Read the model definition and answer for the solid it produces. Units are mm, in the model's axes. A direction names the side the tool comes from. Round coordinates to 2 decimals unless told otherwise and drop trailing zeros. Write each loop counter-clockwise with the first axis right and the second up, starting at its lowest first coordinate (ties: lowest second). Pieces come first, ordered by that corner, then holes. Notation, with made-up numbers: (-37, 57.25) - (-4, 57.25) arc R18 ccw to (-4, 77.25) - close; hole circle Ø7 at (-38, -20.5). An arc over 180 degrees is marked (long way). Use one line per item in the form item = value. Start each with the question number.
1) The part is cut by section D-D, the plane z = 9.5. Give the vertices of the cut face in (x, y), plus the area to 4 significant figures.
2) The part is cut by section A-A, the plane z = 12.5. Give the vertices of the cut face in (x, y), plus the area to 3 significant figures.
3) For faces 1 (the face through (1.25, 3, -8)), 2 (the face through (-8.5, -4, 6)), 3 (the face through (9, -4, 2.45)), 4 (the face through (12, -4, 0)), 5 (the face through (-8.5, -4, -5)), determine the directions among +Z, -Z, +X, -X, +Y, -Y from which every point of the face is accessible in a straight line to the end or side of a thin tool.
4) The part is cut by section C-C, the plane y = 3.75. Give the vertices of the cut face in (x, z), plus the area to 3 significant figures.
5) For a pull along Z with two mould halves and no side action, classify faces 6 (the face through (-10, -8, 0)), 7 (the face through (-11, -4, 0)), 8 (the face through (0, -9, 5)), 9 (the face through (0, -7, 13)) as released by +Z, released by -Z, zero draft, split by the parting line, or undercut.
6) Consider line 1 along X through (y, z) = (-2, 0); line 2 along X through (y, z) = (-8.45, 12.5); line 3 along Y through (x, z) = (-1.5, 11.75). Determine where each line is inside the solid, lowest interval first. Write a range as from..to.
7) Each of these flat-tipped pins is pushed along its axis until it touches: pin 1 (1.2 mm diameter, centred on x = 9, y = -2.5, fed in from +Z); pin 2 (1.3 mm diameter, centred on x = -1, z = 11, fed in from +Y); pin 3 (3 mm diameter, centred on x = -10.1, z = 0, fed in from -Y); pin 4 (1.2 mm diameter, centred on x = -10.05, z = 12.5, fed in from -Y). Where does it stop, or does it pass through?
from build123d import *

# Parameters (mm, degrees)
SKETCH2_R                = 0.9
BOSS_EXTRUDE1_DEPTH      = 8
BOSS_EXTRUDE2_REACH      = 28.314
BOSS_EXTRUDE2_END_RADIUS = 7.55
SKETCH3_W                = 2.5
SKETCH3_H                = 6
SKETCH4_R                = 0.5
CUT_EXTRUDE1_DEPTH       = 8
SKETCH5_W                = 25.1
SKETCH5_H                = 24
BOSS_EXTRUDE3_DEPTH      = 1
SKETCH6_W                = 7.6
SKETCH6_H                = 4.5
BOSS_EXTRUDE4_DEPTH      = 1.5
SKETCH7_R                = 1
CUT_EXTRUDE2_DEPTH       = 31.907118921
SKETCH8_W                = 1.5
SKETCH8_H                = 1
BOSS_EXTRUDE5_DEPTH      = 0.5
SKETCH9_W                = 21
SKETCH9_H                = 5.7
BOSS_EXTRUDE6_DEPTH      = 2.6


with BuildPart() as part:
    # Sketch1 → Revolve1 (revolve)
    with BuildSketch(Plane(origin=(0, 0, 0), x_dir=(0, 0, -1), z_dir=(1, 0, 0))):
        with BuildLine():
            Line((0, 0), (0, 16))
            ThreePointArc((0, 16), (3.744412504, 15.710784808), (7.4, 14.85))
            Line((7.4, 14.85), (8.6, 14.85))
            Line((8.6, 14.85), (8.6, 11.1))
            Line((8.6, 11.1), (8, 11.1))
            Line((8, 11.1), (8, 9.6))
            Line((8, 9.6), (5.9, 9.6))
            Line((5.9, 9.6), (5.9, 6))
            Line((5.9, 6), (7.55, 6))
            Line((7.55, 6), (7.55, 0))
            Line((7.55, 0), (0, 0))
        make_face()
    revolve(axis=Axis((0, 0, 0), (0, 1, 0)))

    # Sketch2 → Boss-Extrude1 (add)
    with BuildSketch(Plane.XZ):
        with BuildLine():
            Line((-8.5, -8.5), (8.5, -8.5))
            Line((8.5, -8.5), (8.5, -2.45))
            Line((8.5, -2.45), (9.55, -2.45))
            ThreePointArc((9.55, -2.45), (12, 0), (9.55, 2.45))
            Line((9.55, 2.45), (8.5, 2.45))
            Line((8.5, 2.45), (8.5, 8.5))
            Line((8.5, 8.5), (-8.5, 8.5))
            Line((-8.5, 8.5), (-8.5, 2.45))
            Line((-8.5, 2.45), (-9.55, 2.45))
            ThreePointArc((-9.55, 2.45), (-12, 0), (-9.55, -2.45))
            Line((-9.55, -2.45), (-8.5, -2.45))
            Line((-8.5, -2.45), (-8.5, -8.5))
        make_face()
        with Locations(Location((-10.1, 0, 0), (0, 0, 270))):
            Circle(SKETCH2_R, mode=Mode.SUBTRACT)
        with Locations(Location((10.1, 0, 0), (0, 0, 270))):
            Circle(SKETCH2_R, mode=Mode.SUBTRACT)
    extrude(amount=BOSS_EXTRUDE1_DEPTH)

    # Boss-Extrude2: up to this cylinder (the profile starts outside it)
    boss_extrude2_end = Plane(origin=(0, 3, 0), z_dir=(0, -1, 0)) * Cylinder(BOSS_EXTRUDE2_END_RADIUS, 72.728, mode=Mode.PRIVATE)
    # Sketch3 → Boss-Extrude2 (add, up to the surface)
    with BuildSketch(Plane(origin=(0, 0, -8.5), x_dir=(-1, 0, 0), z_dir=(0, 0, -1)), mode=Mode.PRIVATE) as boss_extrude2_sk1:
        with Locations((0, 3)):
            Rectangle(SKETCH3_W, SKETCH3_H)
    boss_extrude2_tool1 = extrude(boss_extrude2_sk1.sketch, amount=-BOSS_EXTRUDE2_REACH, mode=Mode.PRIVATE) - boss_extrude2_end
    add(boss_extrude2_tool1.solids().sort_by_distance((0, 3, -8.5))[0])

    # Sketch4 → Cut-Extrude1 (cut)
    with BuildSketch(Plane(origin=(0, 0, -8.5), x_dir=(-1, 0, 0), z_dir=(0, 0, -1))):
        with Locations((0, 3.75)):
            Circle(SKETCH4_R)
    extrude(amount=-CUT_EXTRUDE1_DEPTH, mode=Mode.SUBTRACT)

    # Sketch5 → Boss-Extrude3 (add)
    with BuildSketch(Plane.XZ.offset(8)):
        with Locations((0.45, 2.5)):
            Rectangle(SKETCH5_W, SKETCH5_H)
    extrude(amount=BOSS_EXTRUDE3_DEPTH)

    # Sketch6 → Boss-Extrude4 (add)
    with BuildSketch(Plane(origin=(0, -8, 0), x_dir=(1, 0, 0), z_dir=(0, 1, 0))):
        with Locations((0.2, -10.75)):
            Rectangle(SKETCH6_W, SKETCH6_H)
    extrude(amount=BOSS_EXTRUDE4_DEPTH)

    # Sketch7 → Cut-Extrude2 (cut, through all)
    with BuildSketch(Plane(origin=(0, -8, 0), x_dir=(1, 0, 0), z_dir=(0, 1, 0))):
        with Locations(Location((-10.05, -12.5, 0), (0, 0, 270))):
            Circle(SKETCH7_R)
        with Locations(Location((10.95, -12.5, 0), (0, 0, 270))):
            Circle(SKETCH7_R)
    extrude(amount=-CUT_EXTRUDE2_DEPTH, mode=Mode.SUBTRACT)

    # Sketch8 → Boss-Extrude5 (add)
    with BuildSketch(Plane(origin=(0, -8, 0), x_dir=(1, 0, 0), z_dir=(0, 1, 0))):
        with Locations((-7.65, -9.5)):
            Rectangle(SKETCH8_W, SKETCH8_H)
    extrude(amount=BOSS_EXTRUDE5_DEPTH)

    # Sketch9 → Boss-Extrude6 (add)
    with BuildSketch(Plane.XZ.offset(9)):
        with Locations((0.45, -6.65)):
            Rectangle(SKETCH9_W, SKETCH9_H)
    extrude(amount=BOSS_EXTRUDE6_DEPTH)


solid = part.part
Geometry results:
q1.outline = (-12.1, -9) - (13, -9) - (13, -8) - (4, -8) - (4, -6.5) - (-3.6, -6.5) - (-3.6, -8) - (-6.9, -8) - (-6.9, -7.5) - (-8.4, -7.5) - (-8.4, -8) - (-12.1, -8) - close
q1.area = 37.25 mm2
q2.outline = (-12.1, -9) - (-11.05, -9) - (-11.05, -8) - (-12.1, -8) - close; (-9.05, -9) - (9.95, -9) - (9.95, -8) - (4, -8) - (4, -6.5) - (-3.6, -6.5) - (-3.6, -8) - (-9.05, -8) - close; (11.95, -9) - (13, -9) - (13, -8) - (11.95, -8) - close
q2.area = 32.5 mm2
q3.face_1 = -Z, +X
q3.face_2 = +Z, -X, +Y
q3.face_3 = +Z, +X, +Y
q3.face_4 = +X, +Y
q3.face_5 = -Z, -X, +Y
q4.outline = (-1.25, -8.5) - (-0.5, -8.5) - (-0.5, -0.5) - (0.5, -0.5) - (0.5, -8.5) - (1.25, -8.5) - (1.25, -7.45) arc R7.55 ccw (long way) to (-1.25, -7.45) - close
q4.area = 174 mm2
q5.face_6 = undercut
q5.face_7 = undercut
q5.face_8 = zero draft
q5.face_9 = released by +Z
q6.line_1 = -12..-11, -9.2..9.2, 11..12
q6.line_2 = -12.1..-11.05, -9.05..9.95, 11.95..13
q6.line_3 = -9..-6.5
q7.pin_1 = 8.5
q7.pin_2 = -6.5
q7.pin_3 = -9
q7.pin_4 = through
